For this review, take the finished solid that the model builds, in its own axes (mm). A direction names the side the tool comes from. Give positions to 0.01 mm unless a question says otherwise; leave off trailing zeros. Write each loop counter-clockwise with the first axis right and the second up, starting at its lowest first coordinate (ties: lowest second). Pieces come first, ordered by that corner, then holes. Notation, with made-up numbers: (1.5, 43.25) -> (29.5, 43.25) arc R11 ccw to (29.5, 60.25) -> close; hole circle Ø9 at (44.5, -12). An arc over 180 degrees is marked (long way). Write item = value, one per line.
```python
from build123d import *

# Parameters (mm, degrees)
SKETCH2_R           = 150
BOSS_EXTRUDE1_DEPTH = 6
SKETCH3_R           = 52.5
SKETCH3_R_2         = 50
BOSS_EXTRUDE2_DEPTH = 100
SKETCH4_R           = 5
CUT_EXTRUDE1_DEPTH  = 100


with BuildPart() as part:
    # Sketch2 → Boss-Extrude1 (new body)
    with BuildSketch(Plane.XY):
        Circle(SKETCH2_R)
    extrude(amount=BOSS_EXTRUDE1_DEPTH)

    # Sketch3 → Boss-Extrude2 (add)
    with BuildSketch(Plane.XY.offset(6)):
        Circle(SKETCH3_R)
        Circle(SKETCH3_R_2, mode=Mode.SUBTRACT)
    extrude(amount=BOSS_EXTRUDE2_DEPTH)

    # Sketch4 → Cut-Extrude1 (cut)
    with BuildSketch(Plane.XY.offset(6)):
        with Locations((100, 0)):
            Circle(SKETCH4_R)
        with Locations((0, -100)):
            Circle(SKETCH4_R)
        with Locations((-100, 0)):
            Circle(SKETCH4_R)
        with Locations((0, 100)):
            Circle(SKETCH4_R)
    extrude(amount=-CUT_EXTRUDE1_DEPTH, mode=Mode.SUBTRACT)


solid = part.part
```
(1) For pin 1 (5 mm diameter, centred on x = -118, y = 9, fed in from +Z); pin 2 (6 mm diameter, centred on y = -33.5, z = 90, fed in from -X); pin 3 (6 mm diameter, centred on x = 27.5, z = 91, fed in from -Y), all flat-tipped, find the tip position at first contact; note any pin that passes through.
Answers below:
pin_1 = 6
pin_2 = -42.73
pin_3 = -46.43
(2) The part is to be moulded in two halves that separate along X. For faces 1 (the face through (-95.381, -1.915, 3.042)), 2 (the face through (-19.527, 148.724, 2.958)), 3 (the face through (-1.08, -104.88, 3.04)), 4 (the face through (-2, 2, 0)), say which applies: released by +X, released by -X, zero draft, split by the parting line, or undercut.
Answers below:
face_1 = undercut
face_2 = split by the parting line
face_3 = undercut
face_4 = zero draft
(3) To check wall thickness, follow probe 1 along Y at (x, z) = (0, 4.75); probe 2 along Z at (x, y) = (94.5, -79); probe 3 along Y at (x, z) = (-7.5, 73). State the ranges of each line that lie inside material, in increasing order.
Answers below:
probe_1 = -150 to -105, -95 to 95, 105 to 150
probe_2 = 0 to 6
probe_3 = -51.96 to -49.43, 49.43 to 51.96
(4) Tool access review of faces 5 (the face through (47.69, 15.02, 55.3)), 6 (the face through (-1.08, 95.12, 3.04)): name each direction out of +Z, -Z, +X, -X, +Y, -Y from which nothing blocks a thin tool from reaching the whole face with its end or side.
Answers below:
face_5 = +Z
face_6 = +Z, -Z
(5) Take a section at A-A (y = 0). Write out the cut boundary in (x, z), plus the area to 3 significant figures.
Answers below:
outline = (-150, 0) -> (-105, 0) -> (-105, 6) -> (-150, 6) -> close; (-95, 0) -> (95, 0) -> (95, 6) -> (52.5, 6) -> (52.5, 106) -> (50, 106) -> (50, 6) -> (-50, 6) -> (-50, 106) -> (-52.5, 106) -> (-52.5, 6) -> (-95, 6) -> close; (105, 0) -> (150, 0) -> (150, 6) -> (105, 6) -> close
area = 2,180 mm^2
(6) Take a section at C-C (z = 85). Write out the cut boundary in (x, y).
Answers below:
outline = circle Ø105 at (0, 0); hole circle Ø100 at (0, 0)
(7) Take a section at B-B (x = 100). Write out the cut boundary in (y, z).
Answers below:
outline = (-111.8, 0) -> (-5, 0) -> (-5, 6) -> (-111.8, 6) -> close; (5, 0) -> (111.8, 0) -> (111.8, 6) -> (5, 6) -> close
